```python
from build123d import *

# Parameters (mm, degrees)
SALIENTE_EXTRUIR2_DEPTH      = 11
SALIENTE_EXTRUIR2_DEPTH_BACK = 11
CROQUIS4_R                   = 6
CROQUIS4_R_2                 = 1.7
CORTAR_EXTRUIR2_DEPTH        = 33
CROQUIS5_R                   = 8.2
CORTAR_EXTRUIR3_DEPTH        = 9
CROQUIS6_W                   = 30.6
CROQUIS6_H                   = 7
CORTAR_EXTRUIR4_DEPTH        = 4
CORTAR_EXTRUIR6_DEPTH        = 14
CROQUIS9_R                   = 2.6
CORTAR_EXTRUIR7_DEPTH        = 5


with BuildPart() as part:
    # Croquis2 → Saliente-Extruir2 (new body, two sides)
    with BuildSketch(Plane.XY) as saliente_extruir2_sk:
        with BuildLine():
            Line((-15, -1.5), (-15, 1.5))
            Line((-15, 1.5), (-15, 11.5))
            ThreePointArc((-15, 11.5), (-13.535533906, 15.035533906), (-10, 16.5))
            Line((-10, 16.5), (10, 16.5))
            ThreePointArc((10, 16.5), (13.535533906, 15.035533906), (15, 11.5))
            Line((15, 11.5), (15, 1.5))
            Line((15, 1.5), (15, -1.5))
            Line((15, -1.5), (15, -11.5))
            ThreePointArc((15, -11.5), (13.535533906, -15.035533906), (10, -16.5))
            Line((10, -16.5), (-10, -16.5))
            ThreePointArc((-10, -16.5), (-13.535533906, -15.035533906), (-15, -11.5))
            Line((-15, -11.5), (-15, -1.5))
        make_face()
    extrude(amount=SALIENTE_EXTRUIR2_DEPTH)
    extrude(saliente_extruir2_sk.sketch, amount=-SALIENTE_EXTRUIR2_DEPTH_BACK)

    # Croquis4 → Cortar-Extruir2 (cut)
    with BuildSketch(Plane(origin=(0, 0, -11), x_dir=(-1, 0, 0), z_dir=(0, 0, -1))):
        Circle(CROQUIS4_R)
        with Locations((-11, 0)):
            Circle(CROQUIS4_R_2)
        with Locations((11, 0)):
            Circle(CROQUIS4_R_2)
    extrude(amount=-CORTAR_EXTRUIR2_DEPTH, mode=Mode.SUBTRACT)

    # Croquis5 → Cortar-Extruir3 (cut)
    with BuildSketch(Plane.XY.offset(11)):
        Circle(CROQUIS5_R)
    cortar_extruir3 = extrude(amount=-CORTAR_EXTRUIR3_DEPTH, mode=Mode.SUBTRACT)

    # Croquis6 → Cortar-Extruir4 (cut)
    with BuildSketch(Plane.XY.offset(11)):
        Rectangle(CROQUIS6_W, CROQUIS6_H)
    cortar_extruir4 = extrude(amount=-CORTAR_EXTRUIR4_DEPTH, mode=Mode.SUBTRACT)

    # Croquis8 → Cortar-Extruir6 (cut)
    with BuildSketch(Plane(origin=(0, 0, 0), x_dir=(1, 0, 0), z_dir=(0, 1, 0))):
        Polygon((5, 0), (2.5, 4.330127019), (-2.5, 4.330127019), (-5, 0), (-2.5, -4.330127019), (2.5, -4.330127019), align=None)
    extrude(amount=-CORTAR_EXTRUIR6_DEPTH, mode=Mode.SUBTRACT)

    # Croquis9 → Cortar-Extruir7 (cut)
    with BuildSketch(Plane.XZ.offset(16.5)):
        Circle(CROQUIS9_R)
    extrude(amount=-CORTAR_EXTRUIR7_DEPTH, mode=Mode.SUBTRACT)

    # Simetr_a1: Cortar-Extruir3, Cortar-Extruir4 across plane
    add(cortar_extruir3.mirror(Plane.XY), mode=Mode.SUBTRACT)
    add(cortar_extruir4.mirror(Plane.XY), mode=Mode.SUBTRACT)


solid = part.part
```
Work out the finished part from the listing and answer in its coordinate system (mm). A direction names the side the tool comes from. Give positions to 0.01 mm unless a question says otherwise; leave off trailing zeros. Loops run counter-clockwise (first coordinate to the right, second up) from the corner with the lowest first, then second, coordinate; pieces in that order, holes last. Notation, with made-up numbers: (27.25, 32) - (69.25, 32) arc R10 cw to (69.25, 36) - close; hole circle Ø4 at (85.5, -40). An arc over 180 degrees is marked (long way). Use CSV: the item, a comma, the result in double quotes. Start each with the question number.
(1) Find section B-B, the plane x = 0. Determine the outline of the cut face in (y, z), plus the area to 3 significant figures.
(2) Find the intervals of material crossed by L1, parallel to Y at x = 0, z = -7; L2, parallel to Z at x = 0, y = -15.9; L3, parallel to Z at x = -2, y = -11.5, in increasing order.
(3) Find section C-C, the plane y = 3. Determine the outline of the cut face in (x, z), plus the area to 3 significant figures.
(4) Find section D-D, the plane z = -9.25. Determine the outline of the cut face in (x, y).
(5) Each of these flat-tipped pins is pushed along its axis until it touches: pin 1 (5.5 mm diameter, centred on x = -11, y = 0, fed in from -Z); pin 2 (2 mm diameter, centred on x = -13, z = -9.5, fed in from -Y); pin 3 (3 mm diameter, centred on x = -12.5, z = -8.5, fed in from +Y). Where does it stop, or does it pass through?
(6) Determine the mould class of faces 1 (the face through (11, -3.5, 9)), 2 (the face through (4.045, -9.771, -1.654)), 3 (the face through (13.57, -15, 0.15)), 4 (the face through (-4.01, -9.771, -1.714)) for opening direction X: released by +X, released by -X, zero draft, split by the parting line, or undercut.
(7) Find section A-A, the plane z = 6.25. Determine the outline of the cut face in (x, y), plus the area to 3 significant figures.
(8) A tool of negligible diameter and unlimited length cuts with its end or side. For faces 5 (the face through (-0.338, -15.268, 2.578)), 6 (the face through (4.01, -9.771, 1.714)), 7 (the face through (11, -3.5, -9)), from which of +Z, -Z, +X, -X, +Y, -Y can it reach the whole face along a straight path? Write none if from no direction.
Results found:
1,outline,"(-16.5, -11) - (-8.2, -11) - (-8.2, -4.33) - (-14, -4.33) - (-14, -2.6) - (-16.5, -2.6) - close; (-16.5, 2.6) - (-14, 2.6) - (-14, 4.33) - (-8.2, 4.33) - (-8.2, 11) - (-16.5, 11) - close; (6, -2) - (8.2, -2) - (8.2, -11) - (16.5, -11) - (16.5, 11) - (8.2, 11) - (8.2, 2) - (6, 2) - close"
1,area,"311 mm^2"
2,L1,"-16.5 to -8.2, 8.2 to 16.5"
2,L2,"-11 to -2.6, 2.6 to 11"
2,L3,"-11 to -4.33, 4.33 to 11"
3,outline,"(-15, -7) - (-7.63, -7) - (-7.63, -2) - (-5.2, -2) - (-5.2, 2) - (-7.63, 2) - (-7.63, 7) - (-15, 7) - close; (5.2, -2) - (7.63, -2) - (7.63, -7) - (15, -7) - (15, 7) - (7.63, 7) - (7.63, 2) - (5.2, 2) - close"
3,area,"226 mm^2"
4,outline,"(-15, -11.5) arc R5 ccw to (-10, -16.5) - (10, -16.5) arc R5 ccw to (15, -11.5) - (15, -3.5) - (7.42, -3.5) arc R8.2 cw to (-7.42, -3.5) - (-15, -3.5) - close; (-15, 3.5) - (-7.42, 3.5) arc R8.2 cw to (7.42, 3.5) - (15, 3.5) - (15, 11.5) arc R5 ccw to (10, 16.5) - (-10, 16.5) arc R5 ccw to (-15, 11.5) - close"
5,pin 1,"z = -7"
5,pin 2,"y = -16.08"
5,pin 3,"y = 16.4"
6,face 1,"zero draft"
6,face 2,"undercut"
6,face 3,"released by +X"
6,face 4,"undercut"
7,outline,"(-15, -11.5) arc R5 ccw to (-10, -16.5) - (10, -16.5) arc R5 ccw to (15, -11.5) - (15, 11.5) arc R5 ccw to (10, 16.5) - (-10, 16.5) arc R5 ccw to (-15, 11.5) - close; hole circle Ø3.4 at (-11, 0); hole circle Ø16.4 at (0, 0); hole circle Ø3.4 at (11, 0)"
7,area,"739 mm^2"
8,face 5,"-Y"
8,face 6,"none"
8,face 7,"-Z, +X, -X"
